Here's the drawing with two shaded views (mm, measured from the low corner). I have some questions. A direction names the side the tool comes from. Coordinates: 2 decimals unless noted, no trailing zeros. Order: outer loops, then holes, each group sorted by start corner. A loop starts at its lowest first (then second) coordinate and runs counter-clockwise, first axis right, second up. Notation, with made-up numbers: M 31,56.5 L 69,56.5 A30 cw 69,79.5 Z; hole C -6,73.5 d7. An arc over 180 degrees is marked long. Put each result on its own line as item: value. Start each with the question number.
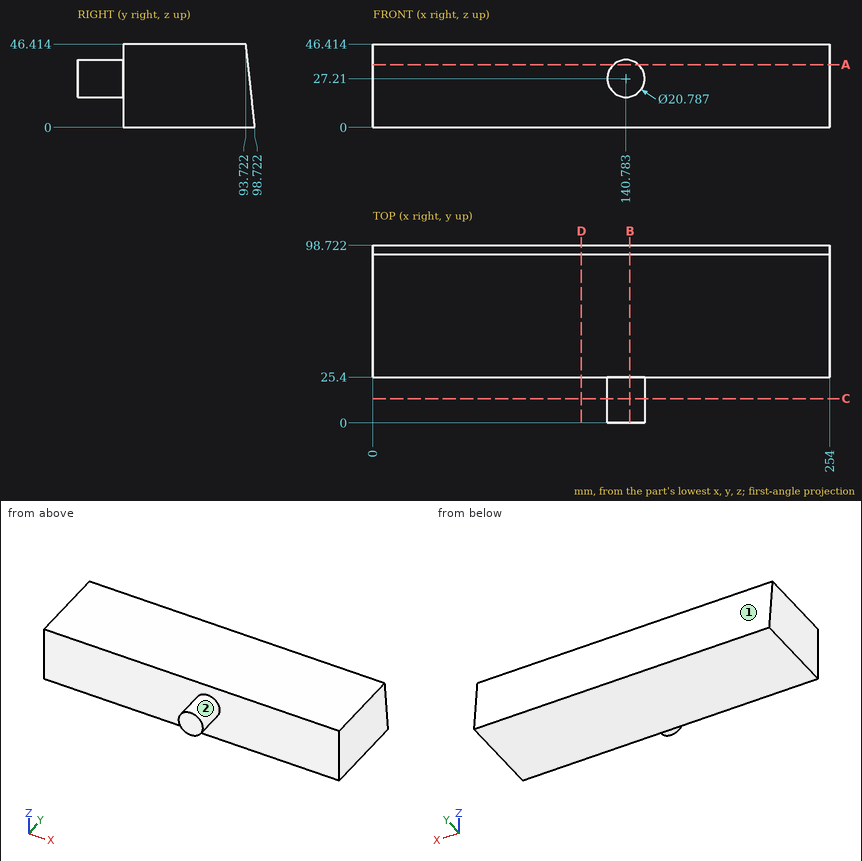
Item 1: If we section it at D-D on x = 116: Write out the boundary of the cut face in (y, z) (1 decimal).
Item 2: If we section it at A-A on z = 35: Write out the boundary of the cut face in (x, y), then the cut area to 3 significant figures.
Item 3: If we section it at B-B on x = 143: Write out the boundary of the cut face in (y, z) (1 decimal), then the cut area to 3 significant figures.
Item 4: I need wall thicknesses on probe 1 along X at (y, z) = (22, 26.5); probe 2 along Y at (x, z) = (104.5, 4); probe 3 along Y at (x, z) = (31, 20). Which ranges of each line are inside material? Lowest first, please.
Item 5: For the marked faces 1 and 2, which set-ups out of +Z, -Z, +X, -X, +Y, -Y let a thin tool reach every point of the face, with its end or its side?
Item 6: For pin 1 Ø1.5 at (x, z) = (160, 17.5) entering from -Y; pin 2 Ø3 at (x, z) = (53, 32.5) entering from +Y; pin 3 Ø1 at (x, z) = (219, 6.5) entering from +Y (1 decimal), each with a flat end and sliding along its axis, tell me the tip position at first contact or that it passes through.
Item 7: If we section it at C-C on y = 13.5: Write out the boundary of the cut face in (x, z), then the cut area to 3 significant figures.
Geometry check:
1. outline: M 25.4,0 L 98.7,0 L 93.7,46.4 L 25.4,46.4 Z
2. outline: M 0,25.4 L 133.9,25.4 L 133.9,0 L 147.66,0 L 147.66,25.4 L 254,25.4 L 254,94.95 L 0,94.95 Z
2. area: 18,000 mm²
3. outline: M 0,17.1 L 25.4,17.1 L 25.4,0 L 98.7,0 L 93.7,46.4 L 25.4,46.4 L 25.4,37.4 L 0,37.4 Z
3. area: 3,800 mm²
4. probe 1: x = 130.41 to 151.15
4. probe 2: y = 25.4 to 98.29
4. probe 3: y = 25.4 to 96.57
5. face 1: +Z, +X, -X, +Y
5. face 2: -Y
6. pin 1: stops at y = 25.4
6. pin 2: stops at y = 95.38
6. pin 3: stops at y = 98.1
7. outline: C 140.78,27.21 d20.79
7. area: 339 mm²
